```python
from build123d import *

# Parameters (mm, degrees)
F0_R     = 8.73125
F1_DEPTH = 19.05
F2_W     = 127
F2_H     = 101.6000000041
F2_R     = 10.31875
F3_DEPTH = 12.7
F5_W     = 25.4
F5_H     = 121.2828524489
F5_W_2   = 69.85
F5_H_2   = 114.3
F6_DEPTH = 6.35
F7_W     = 12.7
F7_H     = 76.2
F8_DEPTH = 127
F10_D    = 16.66748


with BuildPart() as f1:
    # F0 (on Right) → F1 (new body)
    with BuildSketch(Plane.YZ):
        Polygon((44.45, 63.5), (-44.45, 63.5), (-266.8735152621, 152.4009127194), (-368.4735152621, 152.4), (-368.4735152621, -152.4), (-266.8735152621, -152.4009127194), (-44.45, -63.5), (44.45, -63.5), align=None)
        with Locations((-19.05, -38.1)):
            Circle(F0_R, mode=Mode.SUBTRACT)
        with Locations((19.05, -38.1)):
            Circle(F0_R, mode=Mode.SUBTRACT)
        with Locations((-19.05, 38.1)):
            Circle(F0_R, mode=Mode.SUBTRACT)
        with Locations((19.05, 38.1)):
            Circle(F0_R, mode=Mode.SUBTRACT)
    extrude(amount=F1_DEPTH)

    # F2 (on face) → F3 (join)
    with BuildSketch(Plane(origin=(0, -0.0013691088, 152.4033101543), x_dir=(1, 0, 0), z_dir=(0, -8.9835e-06, 1))):
        with Locations((-63.5, -317.6721461661)):
            Rectangle(F2_W, F2_H)
        with Locations((-88.9, -317.6721461661)):
            Circle(F2_R, mode=Mode.SUBTRACT)
    extrude(amount=-F3_DEPTH)

    # F4: F1 across plane


with BuildPart() as f1_1:
    add(f1.part)
    add(f1.part.mirror(Plane.XY))

    # F5 (on Top) → F6 (join, symmetric)
    with BuildSketch(Plane.XY):
        with Locations((-12.7, -295.1320890376)):
            Rectangle(F5_W, F5_H)
        Polygon((-25.4, -234.4906628132), (0, -234.4906628132), (0, -177.8), (-69.85, -177.8), align=None)
        with Locations((-34.925, -120.65)):
            Rectangle(F5_W_2, F5_H_2)
    extrude(amount=F6_DEPTH, both=True)

    # F7 (on face) → F8 (join)
    with BuildSketch(Plane(origin=(0, 0, 0), x_dir=(0, -1, 0), z_dir=(-1, 0, 0))):
        with Locations((57.15, 0)):
            Rectangle(F7_W, F7_H)
    extrude(amount=F8_DEPTH)

    # F10 (through all)
    with Locations(Plane(origin=(0, -50.8, 0), x_dir=(-1, 0, 0), z_dir=(0, 1, 0))):
        with Locations((88.9, 19.05), (88.9, -19.05)):
            Hole(F10_D / 2)


solid = f1_1.part
```
Geometry: final body of the model. Coordinates: model frame, mm. A direction names the side the tool comes from. Coordinates: 2 decimals unless noted, no trailing zeros. Order: outer loops, then holes, each group sorted by start corner. A loop starts at its lowest first (then second) coordinate and runs counter-clockwise, first axis right, second up.
Item 1: Section query B-B (x = -6.5). Output: boundary loops of the cut face in (y, z).
Answer:
outline: (-368.47, -152.4) - (-266.87, -152.4) - (-266.87, -139.7) - (-368.47, -139.7) - close; (-368.47, 139.7) - (-266.87, 139.7) - (-266.87, 152.4) - (-368.47, 152.4) - close; (-355.77, -6.35) - (-63.5, -6.35) - (-63.5, -38.1) - (-50.8, -38.1) - (-50.8, 38.1) - (-63.5, 38.1) - (-63.5, 6.35) - (-355.77, 6.35) - close
Item 2: Access query for faces 4 (the face through (-28, -175, 6.35)), 5 (the face through (9, 1, 63.5)), 6 (the face through (-63, -50.8, -1)). Directions: +Z, -Z, +X, -X, +Y, -Y. A direction counts if a zero-diameter tool reaches every point of the face in a straight line with its end or side. Return the directions, or none.
Answer:
face 4: -X, -Y
face 5: +Z, +X, -X, +Y
face 6: +Z, -Z, -X, +Y
Item 3: Section query A-A (y = -19.05). Output: boundary loops of the cut face in (x, z).
Answer:
outline: (0, -63.5) - (19.05, -63.5) - (19.05, -46.83) - (0, -46.83) - close; (0, -29.37) - (19.05, -29.37) - (19.05, 29.37) - (0, 29.37) - close; (0, 46.83) - (19.05, 46.83) - (19.05, 63.5) - (0, 63.5) - close
Item 4: Contact query for flat-ended pins moving along their axis: P1, Ø15, axis at x = 14.5, y = -22, coming from the +Z side; P2, Ø1, axis at y = -69.5, z = -54, coming from the -X side; P3, Ø14, axis at y = -103, z = -2, coming from the -X side. Output: stop coordinate, or through.
Answer:
P1: stops at z = 63.5
P2: stops at x = 0
P3: stops at x = -69.85
Item 5: Section query C-C (z = 19.05). Output: boundary loops of the cut face in (x, y).
Answer:
outline: (-127, -63.5) - (-97.23, -63.5) - (-97.23, -50.8) - (-127, -50.8) - close; (-80.57, -63.5) - (0, -63.5) - (0, -368.47) - (19.05, -368.47) - (19.05, 44.45) - (0, 44.45) - (0, -50.8) - (-80.57, -50.8) - close
Item 6: Material intervals for line 1 along Z through (x, y) = (13.5, 19.05); line 2 along Z through (x, y) = (-88.9, -59.25); line 3 along Y through (x, z) = (-88.9, 144.5), sorted ascending.
Answer:
line 1: z = -63.5 to -46.83, -29.37 to 29.37, 46.83 to 63.5
line 2: z = -38.1 to -27.38, -10.72 to 10.72, 27.38 to 38.1
line 3: y = -368.47 to -327.99, -307.35 to -266.87
Item 7: Draft query along Y for faces 1 (the face through (-25.4, -296, 0)), 2 (the face through (9.392, -157.219, -108.573)), 3 (the face through (9.39, -10.72, 40.72)). Return one class per face: released by +Y, released by -Y, zero draft, split by the parting line, or undercut.
Answer:
face 1: zero draft
face 2: released by +Y
face 3: undercut
Item 8: Section query D-D (x = -88.9). Output: boundary loops of the cut face in (y, z), then the cut area to 3 significant figures.
Answer:
outline: (-368.47, -152.4) - (-327.99, -152.4) - (-327.99, -139.7) - (-368.47, -139.7) - close; (-368.47, 139.7) - (-327.99, 139.7) - (-327.99, 152.4) - (-368.47, 152.4) - close; (-307.35, -152.4) - (-266.87, -152.4) - (-266.87, -139.7) - (-307.35, -139.7) - close; (-307.35, 139.7) - (-266.87, 139.7) - (-266.87, 152.4) - (-307.35, 152.4) - close; (-63.5, -38.1) - (-50.8, -38.1) - (-50.8, -27.38) - (-63.5, -27.38) - close; (-63.5, -10.72) - (-50.8, -10.72) - (-50.8, 10.72) - (-63.5, 10.72) - close; (-63.5, 27.38) - (-50.8, 27.38) - (-50.8, 38.1) - (-63.5, 38.1) - close
area: 2,600 mm2
